Input: part model. Units: mm. Frame: model coordinates. Coordinates: 2 decimals unless noted, no trailing zeros. Order: outer loops, then holes, each group sorted by start corner. A loop starts at its lowest first (then second) coordinate and runs counter-clockwise, first axis right, second up.
Solid Edge part; units mm, degrees
sketch "Sketch1" plane through (0, 0, 0) normal (0, 0, 1) x (1, 0, 0)
  circle A0 centre (0, 0) radius 47.625
extrude "Protrusion1" add sketch "Sketch1" along normal blind 12.7
sketch "Sketch2" plane through (0, 0, 12.7) normal (0, 0, 1) x (1, 0, 0)
  circle A0 centre (0, 0) radius 50.8
  circle A1 centre (0, 0) radius 47.625
extrude "ExtrudedProtrusion_3" add sketch "Sketch2" against normal blind 12.7
hole "Hole_1" at (0, 0, 12.7) direction (0, 0, -1) diameter 6.35 end up to next
properties part number "SPaRC - 01 - 002"
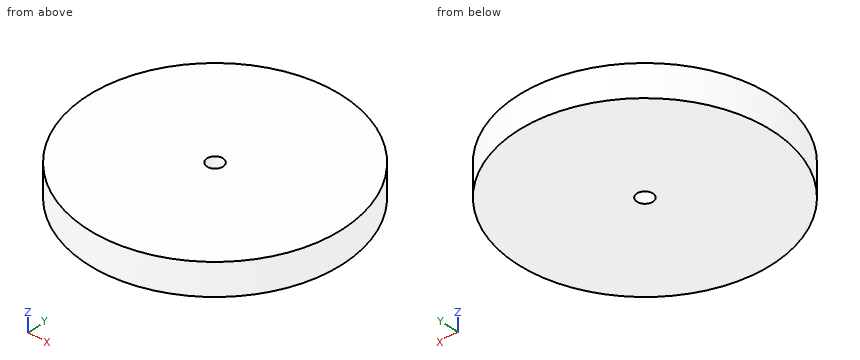
Item 1: Cut plane C-C on z = 8.5. Return loops of the section in (x, y) (3 decimals), then the cut area to 3 significant figures.
Response values:
outline: circle Ø101.6 at (0, 0); hole circle Ø6.35 at (0, 0)
area: 8,080 mm2
Item 2: Ray query, probe 1 along Y at (x, z) = (0, 9.75) (3 decimals); probe 2 along Y at (x, z) = (32, 5); probe 3 along Y at (x, z) = (23.5, 9). Return the intervals inside material, ascending.
Response values:
probe 1: y = -50.8 to -3.175, 3.175 to 50.8
probe 2: y = -39.45 to 39.45
probe 3: y = -45.04 to 45.04
Item 3: Cut plane A-A on y = 0. Return loops of the section in (x, z) (3 decimals), then the cut area to 3 significant figures.
Response values:
outline: (-50.8, 0) - (-3.175, 0) - (-3.175, 12.7) - (-50.8, 12.7) - close; (3.175, 0) - (50.8, 0) - (50.8, 12.7) - (3.175, 12.7) - close
area: 1,210 mm2
Item 4: Pin query (flat end, axial travel): pin 1 Ø1 at (x, z) = (15.5, 2) entering from -Y; pin 2 Ø6 at (x, z) = (31, 3) entering from +Y; pin 3 Ø1.5 at (y, z) = (-30.5, 8) entering from +X. Return the tip coordinate at first contact, or that it passes through.
Response values:
pin 1: stops at y = -48.53
pin 2: stops at y = 42.39
pin 3: stops at x = 41.18
Item 5: Cut plane D-D on x = -24. Return loops of the section in (y, z), then the cut area to 3 significant figures.
Response values:
outline: (-44.77, 0) - (44.77, 0) - (44.77, 12.7) - (-44.77, 12.7) - close
area: 1,140 mm2
